CAD build for the part. Positions are in the model's coordinates, mm. Face numbers are marked on the shaded views. A direction names the side the tool comes from. Round coordinates to 2 decimals unless told otherwise and drop trailing zeros. Order: outer loops, then holes, each group sorted by start corner. A loop starts at its lowest first (then second) coordinate and runs counter-clockwise, first axis right, second up. Notation, with made-up numbers: M -25,-22 L 33,-22 A21 cw 33,-7 Z; hole C -12,2 d2. An arc over 180 degrees is marked long. Answer as a JSON object with one key per item and string values.
```python
from build123d import *

# Parameters (mm, degrees)
SKETCH1_W           = 152.4
SKETCH1_H           = 152.4
SKETCH1_R           = 64.008
BOSS_EXTRUDE1_DEPTH = 22.225
SKETCH2_W           = 152.4
SKETCH2_H           = 152.4
BOSS_EXTRUDE2_DEPTH = 6.35
SKETCH3_R           = 2.032
BOSS_EXTRUDE3_DEPTH = 2.54
CIRPATTERN1_COUNT   = 12


with BuildPart() as part:
    # Sketch1 → Boss-Extrude1 (new body)
    with BuildSketch(Plane(origin=(0, 0, 0), x_dir=(1, 0, 0), z_dir=(0, 1, 0))):
        Rectangle(SKETCH1_W, SKETCH1_H)
        Circle(SKETCH1_R, mode=Mode.SUBTRACT)
    extrude(amount=BOSS_EXTRUDE1_DEPTH)

    # Sketch2 → Boss-Extrude2 (add)
    with BuildSketch(Plane(origin=(0, 0, 0), x_dir=(-1, 0, 0), z_dir=(0, -1, 0))):
        Rectangle(SKETCH2_W, SKETCH2_H)
    extrude(amount=BOSS_EXTRUDE2_DEPTH)

    # Sketch3 → Boss-Extrude3 (add)
    with BuildSketch(Plane(origin=(0, 0, 0), x_dir=(1, 0, 0), z_dir=(0, 1, 0))):
        with Locations((-58.42, 0)):
            Circle(SKETCH3_R)
    boss_extrude3 = extrude(amount=BOSS_EXTRUDE3_DEPTH)

    # CirPattern1: Boss-Extrude3 ×12 about axis
    cirpattern1_axis = Axis((0, 0, 0), (0, 1, 0))
    for i in range(1, CIRPATTERN1_COUNT):
        add(boss_extrude3.rotate(cirpattern1_axis, i * 360 / CIRPATTERN1_COUNT))


solid = part.part
```
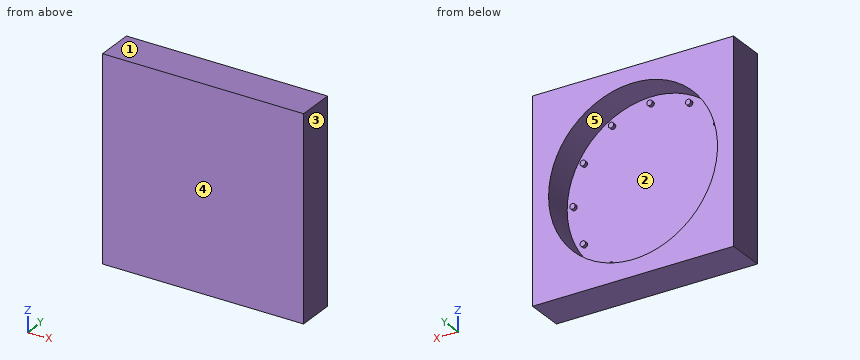
Item 1: Saw through at D-D on z = 58.42. List the corners of the cut face in (x, y) (3 decimals), and give its area (3 significant figures).
Worked answers:
{"outline": "M -76.2,-6.35 L 76.2,-6.35 L 76.2,22.225 L 26.156,22.225 L 26.156,0 L 2.032,0 L 2.032,2.54 L -2.032,2.54 L -2.032,0 L -26.156,0 L -26.156,22.225 L -76.2,22.225 Z", "area": "3,200 mm2"}
Item 2: Saw through at C-C on x = -58.42. List the corners of the cut face in (y, z) (3 decimals).
Worked answers:
{"outline": "M -6.35,-76.2 L 22.225,-76.2 L 22.225,-26.156 L 0,-26.156 L 0,-2.032 L 2.54,-2.032 L 2.54,2.032 L 0,2.032 L 0,26.156 L 22.225,26.156 L 22.225,76.2 L -6.35,76.2 Z"}
Item 3: Drop flat-ended pins along their axis: pin 1 Ø2 at (x, z) = (-28.5, -50.5) entering from +Y; pin 2 Ø5 at (x, z) = (28, 43.5) entering from +Y. Give the stop position or say it passes through.
Worked answers:
{"pin 1": "stops at y = 2.54", "pin 2": "stops at y = 0"}
Item 4: Two-plate mould, pull along X, no slides. Class the marked faces 3, 4 and 5: released by +X, released by -X, zero draft, split by the parting line, or undercut.
Worked answers:
{"face 3": "released by +X", "face 4": "zero draft", "face 5": "undercut"}
Item 5: Saw through at A-A on y = 11.25. List the corners of the cut face in (x, z), and give its area (3 significant figures).
Worked answers:
{"outline": "M -76.2,-76.2 L 76.2,-76.2 L 76.2,76.2 L -76.2,76.2 Z; hole C 0,0 d128.02", "area": "10,400 mm2"}
Item 6: Saw through at B-B on z = 0. List the corners of the cut face in (x, y) (3 decimals).
Worked answers:
{"outline": "M -76.2,-6.35 L 76.2,-6.35 L 76.2,22.225 L 64.008,22.225 L 64.008,0 L 60.452,0 L 60.452,2.54 L 56.388,2.54 L 56.388,0 L -56.388,0 L -56.388,2.54 L -60.452,2.54 L -60.452,0 L -64.008,0 L -64.008,22.225 L -76.2,22.225 Z"}
Item 7: 3-axis set-ups, long thin cutter, end or side, ignore diameter. For the marked faces 1 and 2: which of +Z, -Z, +X, -X, +Y, -Y reach the whole face in a straight line?
Worked answers:
{"face 1": "+Z, +X, -X, +Y, -Y", "face 2": "+Y"}
Item 8: Wall check: line 1 along Z through (x, y) = (0, 10); line 2 along X through (y, z) = (2.25, 54.5). Give the ranges that are in metal, low to high. Write a range as [from, to].
Worked answers:
{"line 1": "z = [-76.2, -64.01], [64.01, 76.2]", "line 2": "x = [-76.2, -33.57], [33.57, 76.2]"}
